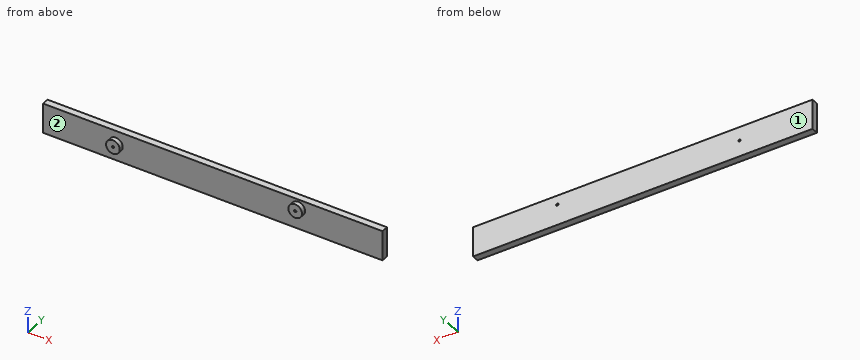
from build123d import *

# Parameters (mm, degrees)
F0_W     = 149
F0_H     = 13
F1_DEPTH = 3
F2_R     = 3
F3_DEPTH = 2
F4_D     = 1


with BuildPart() as f1:
    # F0 (on Front) → F1 (new body)
    with BuildSketch(Plane.XZ):
        with Locations((-4.2446807389, -6.5)):
            Rectangle(F0_W, F0_H)
    extrude(amount=F1_DEPTH)

    # F2 (on face) → F3 (join)
    with BuildSketch(Plane.XZ.offset(3)):
        with Locations((-46.7446807389, -6)):
            Circle(F2_R)
        with Locations((33.2553192611, -4)):
            Circle(F2_R)
    extrude(amount=F3_DEPTH)

    # F4 (through all)
    with Locations(Plane(origin=(0, 0, 0), x_dir=(1, 0, 0), z_dir=(0, 1, 0))):
        with Locations((-46.7446807389, 6), (33.2553192611, 4)):
            Hole(F4_D / 2)


solid = f1.part
Geometry check sheet. Reference: the model listing, model coordinates, mm. Face numbers are marked on the shaded views. Round coordinates to 2 decimals unless told otherwise and drop trailing zeros. Order: outer loops, then holes, each group sorted by start corner. A loop starts at its lowest first (then second) coordinate and runs counter-clockwise, first axis right, second up. Notation, with made-up numbers: M 53,89 L 76,89 A20 cw 76,110 Z; hole C 56,-28 d7. An arc over 180 degrees is marked long. Write each question's results on one line, items separated by ' | '. Start each with the question number.
1. Cross-section at B-B on x = 13. Record the boundary of the cut face in (y, z), plus the area to 3 significant figures.
2. Draft check along X on the marked faces 1 and 2. Enter one of: pulls with the +X half, pulls with the -X half, needs draft (parallel to the pull), parting line crosses it, or undercut.
3. Material ranges on L1, parallel to X at y = -2.05, z = -6; L2, parallel to Y at x = -24, z = -5.25; L3, parallel to X at y = -0.4, z = -3.75, recorded low to high. Write a range as from..to.
4. Cross-section at A-A on z = -11. Record the boundary of the cut face in (x, y), plus the area to 3 significant figures.
Resolved:
1) outline: M -3,-13 L 0,-13 L 0,0 L -3,0 Z | area: 39.0 mm2
2) face 1: needs draft | face 2: undercut
3) L1: -78.74..-47.24, -46.24..70.26 | L2: -3..0 | L3: -78.74..32.82, 33.69..70.26
4) outline: M -78.74,-3 L 70.26,-3 L 70.26,0 L -78.74,0 Z | area: 447 mm2
